Read the model definition and answer for the solid it produces. Units are mm, in the model's axes. Face numbers are marked on the shaded views. A direction names the side the tool comes from. Give positions to 0.01 mm unless a question says otherwise; leave off trailing zeros. Loops run counter-clockwise (first coordinate to the right, second up) from the corner with the lowest first, then second, coordinate; pieces in that order, holes last. Notation, with made-up numbers: (-18, 26) - (-13, 26) arc R9 cw to (-13, 42) - close; hole circle Ø1 at (-29.5, 74.5). An arc over 180 degrees is marked (long way). Put each result on its own line as item: value. Start each with the question number.
1. A cutting plane is placed at D-D, the plane y = 76.5. Determine the outline of the cut face in (x, z), plus the area to 3 significant figures.
2. Consider L1, parallel to X at y = 63, z = 0; L2, parallel to Y at x = -1, z = 15.5; L3, parallel to Y at x = 1.5, z = -6.5. Determine where each line is inside the solid, lowest interval first. Write a range as from..to.
3. A cutting plane is placed at A-A, the plane z = 0. Determine the outline of the cut face in (x, y), plus the area to 4 significant figures.
4. A cutting plane is placed at C-C, the plane y = 62. Determine the outline of the cut face in (x, z).
5. Given pin 1 Ø4 at (y, z) = (34.5, -6.5) entering from -X; pin 2 Ø2 at (x, z) = (14, 0) entering from +Y; pin 3 Ø8 at (y, z) = (51.5, -10) entering from +X, each flat-ended and moving along its own axis, determine where each tip first touches the part or whether it passes through.
6. For the marked faces 1, 2 and 3, determine the directions among +Z, -Z, +X, -X, +Y, -Y from which every point of the face is accessible in a straight line to the end or side of a thin tool.
```python
from build123d import *

# Parameters (mm, degrees)
ESQUISSE1_R                  = 17
BOSS_EXTRU_1_DEPTH           = 43
ESQUISSE2_R                  = 18
BOSS_EXTRU_2_DEPTH           = 22
ESQUISSE3_R                  = 6
BOSS_EXTRU_3_DEPTH           = 5
ESQUISSE4_R                  = 3
BOSS_EXTRU_4_DEPTH           = 25
ESQUISSE5_R                  = 1.25
ENL_V_MAT_EXTRU_1_DEPTH      = 5
ESQUISSE6_W                  = 15
ESQUISSE6_H                  = 5
BOSS_EXTRU_5_DEPTH           = 5
ENL_V_MAT_EXTRU_4_DEPTH      = 10
ENL_V_MAT_EXTRU_4_DEPTH_BACK = 22
ESQUISSE8_R                  = 5
BOSS_EXTRU_6_DEPTH           = 1
ESQUISSE9_R                  = 3.25
BOSS_EXTRU_7_DEPTH           = 4


with BuildPart() as part:
    # Esquisse1 → Boss.-Extru.1 (new body)
    with BuildSketch(Plane(origin=(0, 0, 0), x_dir=(1, 0, 0), z_dir=(0, 1, 0))):
        with Locations(Location((0, 0, 0), (0, 0, 270))):
            Circle(ESQUISSE1_R)
    extrude(amount=BOSS_EXTRU_1_DEPTH)

    # Esquisse2 → Boss.-Extru.2 (add)
    with BuildSketch(Plane(origin=(0, 43, 0), x_dir=(1, 0, 0), z_dir=(0, 1, 0))):
        with Locations(Location((0, 0, 0), (0, 0, 270))):
            Circle(ESQUISSE2_R)
    extrude(amount=BOSS_EXTRU_2_DEPTH)

    # Esquisse3 → Boss.-Extru.3 (add)
    with BuildSketch(Plane(origin=(0, 65, 0), x_dir=(1, 0, 0), z_dir=(0, 1, 0))):
        with Locations(Location((0, 7, 0), (0, 0, 270))):
            Circle(ESQUISSE3_R)
    extrude(amount=BOSS_EXTRU_3_DEPTH)

    # Esquisse4 → Boss.-Extru.4 (add)
    with BuildSketch(Plane(origin=(0, 70, 0), x_dir=(1, 0, 0), z_dir=(0, 1, 0))):
        with Locations(Location((0, 7, 0), (0, 0, 270))):
            Circle(ESQUISSE4_R)
    extrude(amount=BOSS_EXTRU_4_DEPTH)

    # Esquisse5 → Enlèv. mat.-Extru.1 (cut)
    with BuildSketch(Plane(origin=(0, 65, 0), x_dir=(1, 0, 0), z_dir=(0, 1, 0))):
        with Locations(Location((14, 0, 0), (0, 0, 270))):
            Circle(ESQUISSE5_R)
        with Locations(Location((-14, 0, 0), (0, 0, 270))):
            Circle(ESQUISSE5_R)
    extrude(amount=-ENL_V_MAT_EXTRU_1_DEPTH, mode=Mode.SUBTRACT)

    # Esquisse6 → Boss.-Extru.5 (add)
    with BuildSketch(Plane.XZ):
        with Locations((0, -10)):
            Rectangle(ESQUISSE6_W, ESQUISSE6_H)
    extrude(amount=BOSS_EXTRU_5_DEPTH)

    # Esquisse7 → Enlèv. mat.-Extru.4 (cut, two sides)
    with BuildSketch(Plane(origin=(0, 95, 0), x_dir=(1, 0, 0), z_dir=(0, 1, 0))) as enl_v_mat_extru_4_sk:
        with BuildLine():
            Line((-1.8, 9.4), (1.8, 9.4))
            ThreePointArc((1.8, 9.4), (0, 10), (-1.8, 9.4))
        make_face()
    extrude(amount=ENL_V_MAT_EXTRU_4_DEPTH, mode=Mode.SUBTRACT)
    extrude(enl_v_mat_extru_4_sk.sketch, amount=-ENL_V_MAT_EXTRU_4_DEPTH_BACK, mode=Mode.SUBTRACT)

    # Esquisse8 → Boss.-Extru.6 (add)
    with BuildSketch(Plane.XZ):
        with Locations(Location((0, 0, 0), (0, 0, 90))):
            Circle(ESQUISSE8_R)
    extrude(amount=BOSS_EXTRU_6_DEPTH)

    # Esquisse9 → Boss.-Extru.7 (add)
    with BuildSketch(Plane.XZ.offset(1)):
        with Locations(Location((0, 0, 0), (0, 0, 270))):
            Circle(ESQUISSE9_R)
    extrude(amount=BOSS_EXTRU_7_DEPTH)


solid = part.part
```
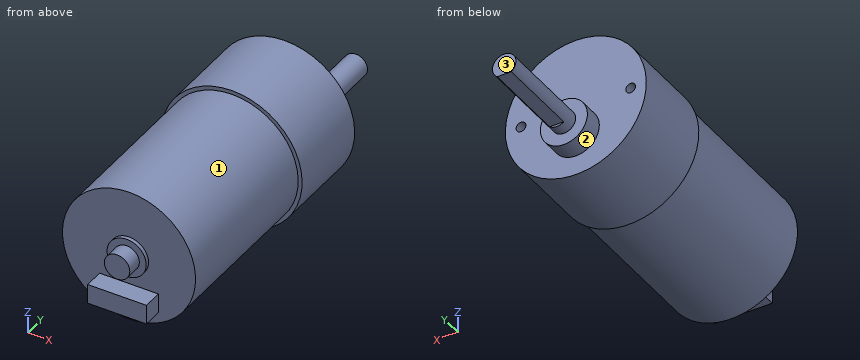
Return value:
1. outline: (-1.8, -9.4) - (1.8, -9.4) arc R3 ccw (long way) to start
1. area: 26.8 mm2
2. L1: x = -18..-15.25, -12.75..12.75, 15.25..18
2. L2: y = 0..65
2. L3: y = 0..95
3. outline: (-18, 43) - (-17, 43) - (-17, 0) - (-5, 0) - (-5, -1) - (-3.25, -1) - (-3.25, -5) - (3.25, -5) - (3.25, -1) - (5, -1) - (5, 0) - (17, 0) - (17, 43) - (18, 43) - (18, 65) - (15.25, 65) - (15.25, 60) - (12.75, 60) - (12.75, 65) - (-12.75, 65) - (-12.75, 60) - (-15.25, 60) - (-15.25, 65) - (-18, 65) - close
3. area: 2,265 mm2
4. outline: circle Ø36 at (0, 0); hole circle Ø2.5 at (-14, 0); hole circle Ø2.5 at (14, 0)
5. pin 1: stops at x = -16.39
5. pin 2: stops at y = 60
5. pin 3: stops at x = 16.97
6. face 1: -Y
6. face 2: +Y
6. face 3: +Z, -Z, +X, -X, +Y
